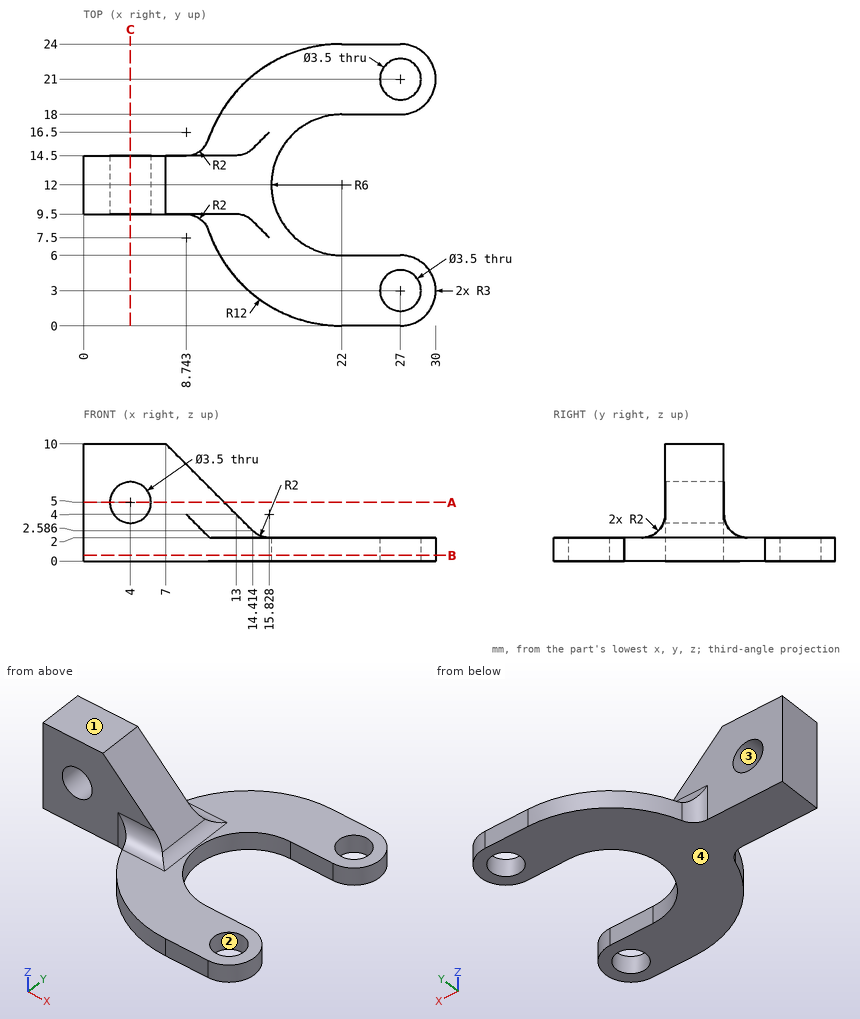
Part print with two shaded views. Sizes in mm from the minimum x, y, z corner. Round coordinates to 2 decimals unless told otherwise and drop trailing zeros. Order: outer loops, then holes, each group sorted by start corner. A loop starts at its lowest first (then second) coordinate and runs counter-clockwise, first axis right, second up. Notation, with made-up numbers: M -22.5,87 L -0.5,87 A9 ccw -0.5,99 Z; hole C -36.75,22.25 d11. An arc over 180 degrees is marked long. Answer in a Markdown table with one row per item. Add a question column.
Q1. Cut at B-B on z = 0.5. Give the cut face in (x, y).
Q2. Pin check, flat tips, straight feed: pin 1 (5.5 mm diameter, centred on x = 27, y = 21, fed in from +Z); pin 2 (3 mm diameter, centred on x = 7, z = 4.5, fed in from -Y); pin 3 (3 mm diameter, centred on y = 5.5, z = 1.5, fed in from -X). Stop position of each tip, or through.
Q3. Cut at C-C on x = 4. Give the cut face in (y, z), and give its area (3 significant figures).
Q4. Mould opens along Z. For the marked faces 1, 2, 3 and 4 say: +Z half, -Z half, draft (parallel to the pull), parting line (faces both ways), or undercut.
Q5. Wall check: L1, parallel to Y at x = 27, z = 1.45; L2, parallel to Y at x = 26, z = 1 (1 decimal); L3, parallel to Z at x = 4, y = 10.9. Give the ranges that are in metal, low to high. Write a range as from..to.
Q6. Cut at A-A on z = 5. Give the cut face in (x, y), and give its area (3 significant figures).
Established:
| question | item | result |
|---|---|---|
| 1 | outline | M 0,9.5 L 8.74,9.5 A2 cw 10.64,8.14 A12 ccw 22,0 L 27,0 A3 ccw 27,6 L 22,6 A6 cw 22,18 L 27,18 A3 ccw 27,24 L 22,24 A12 ccw 10.64,15.86 A2 cw 8.74,14.5 L 0,14.5 Z; hole C 27,3 d3.5; hole C 27,21 d3.5 |
| 2 | pin 1 | stops at z = 2 |
| 2 | pin 2 | stops at y = 9.5 |
| 2 | pin 3 | stops at x = 11.09 |
| 3 | outline | M 9.5,0 L 14.5,0 L 14.5,3.25 L 9.5,3.25 Z; M 9.5,6.75 L 14.5,6.75 L 14.5,10 L 9.5,10 Z |
| 3 | area | 32.5 mm2 |
| 4 | face 1 | +Z half |
| 4 | face 2 | draft |
| 4 | face 3 | undercut |
| 4 | face 4 | -Z half |
| 5 | L1 | y = 0..1.25, 4.75..6, 18..19.25, 22.75..24 |
| 5 | L2 | y = 0..1.6, 4.4..6, 18..19.6, 22.4..24 |
| 5 | L3 | z = 0..3.25, 6.75..10 |
| 6 | outline | M 0,9.5 L 2.25,9.5 L 2.25,14.5 L 0,14.5 Z; M 5.75,9.5 L 12,9.5 L 12,14.5 L 5.75,14.5 Z |
| 6 | area | 42.5 mm2 |
